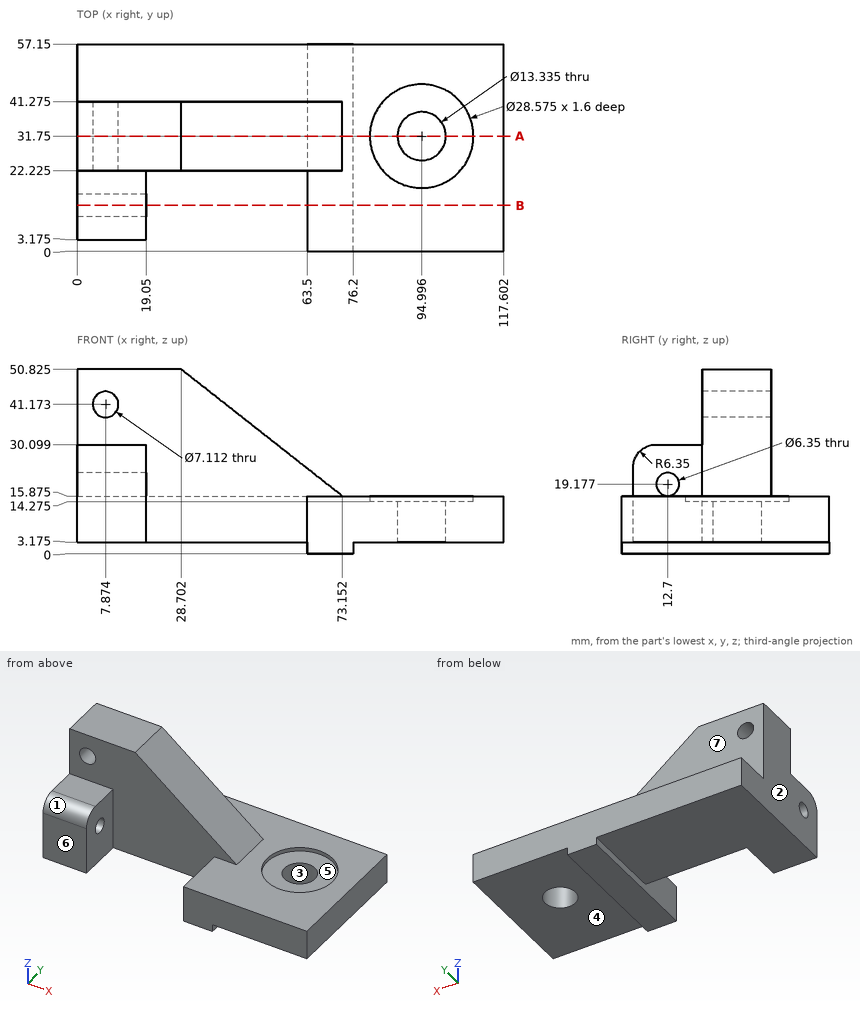
Job drawing, mm, ordinate dimensions from the low corner. One solid piece. A direction names the side the tool comes from. Coordinates: 2 decimals unless noted, no trailing zeros. Order: outer loops, then holes, each group sorted by start corner. A loop starts at its lowest first (then second) coordinate and runs counter-clockwise, first axis right, second up. Notation, with made-up numbers: (-32.75, -22.75) - (22.25, -22.75) arc R28 cw to (22.25, -1.75) - close; hole circle Ø4 at (78, 21.5). An arc over 180 degrees is marked (long way). Write each question's results on one line, items separated by ' | '. Start each with the question number.
Item 1: Band-saw the part on B-B on y = 12.7. State how many separate pieces and enclosed holes the cut face has, and give its area (3 significant figures).
Item 2: Wall check: probe 1 along Y at (x, z) = (23, 20) (1 decimal); probe 2 along Z at (x, y) = (70, 15) (1 decimal); probe 3 along X at (y, z) = (16.5, 11). Give the ranges that are in metal, low to high. Write a range as [from, to].
Item 3: Tool access for the marked faces 4, 5, 6 and 7: list every direction of +Z, -Z, +X, -X, +Y, -Y with a clear straight run to the whole face (end or side of a thin tool).
Item 4: Mould opens along Y. For the marked faces 1, 2 and 3 say: released by +Y, released by -Y, zero draft, split by the parting line, or undercut.
Item 5: Band-saw the part on A-A on y = 31.75. Write the cut outline in (x, z) (1 decimal), and give its area (3 significant figures).
Item 6: Flat gauge pins, fed straight in: pin 1 (3 mm diameter, centred on x = 51.5, y = 28.5, fed in from -Z) (3 decimals); pin 2 (15 mm diameter, centred on x = 5, z = 11, fed in from -Y) (3 decimals); pin 3 (8 mm diameter, centred on x = 27, z = 38, fed in from +Y) (3 decimals); pin 4 (4.5 mm diameter, centred on x = 7.87, z = 41.17, fed in from +Y). Where does each tip first touch, or does it go through?
Numbers:
1) separate pieces: 3 | enclosed holes: 0 | area: 1,120 mm^2
2) probe 1: [22.2, 41.3] | probe 2: [0, 15.9] | probe 3: [0, 19.05], [63.5, 117.6]
3) face 4: -Z, +X, +Y, -Y | face 5: +Z | face 6: +Z, -Z, -X, -Y | face 7: +Z, +X, -X, +Y
4) face 1: released by -Y | face 2: zero draft | face 3: undercut
5) outline: (0, 3.2) - (63.5, 3.2) - (63.5, 0) - (76.2, 0) - (76.2, 3.2) - (88.3, 3.2) - (88.3, 14.3) - (80.7, 14.3) - (80.7, 15.9) - (73.2, 15.9) - (28.7, 50.8) - (0, 50.8) - close; (101.7, 3.2) - (117.6, 3.2) - (117.6, 15.9) - (109.3, 15.9) - (109.3, 14.3) - (101.7, 14.3) - close; hole circle Ø7.1 at (7.9, 41.2) | area: 3,080 mm^2
6) pin 1: z = 3.175 | pin 2: y = 3.175 | pin 3: y = 41.275 | pin 4: through
